Read the model definition and answer for the solid it produces. Units are mm, in the model's axes. A direction names the side the tool comes from. Coordinates: 2 decimals unless noted, no trailing zeros. Write each loop counter-clockwise with the first axis right and the second up, starting at its lowest first coordinate (ties: lowest second). Pieces come first, ordered by that corner, then holes. Notation, with made-up numbers: (-24, -30) -> (23, -30) arc R27 ccw to (23, 2) -> close; hole circle Ø8 at (89.25, 47). An arc over 180 degrees is marked (long way). One line per item, written item: value. Start each with the question number.
from build123d import *

# Parameters (mm, degrees)
RESSALTO_EXTRUS_O1_DEPTH = 5
ESBO_O4_W                = 4.495494134
ESBO_O4_H                = 25
CORTE_EXTRUS_O2_DEPTH    = 5
ESBO_O11_W               = 5
ESBO_O11_H               = 25
CORTE_EXTRUS_O8_DEPTH    = 10
ESBO_O24_W               = 15
ESBO_O24_H               = 60
CORTE_EXTRUS_O14_DEPTH   = 10
ESBO_O27_W               = 15
ESBO_O27_H               = 60
CORTE_EXTRUS_O16_DEPTH   = 25


with BuildPart() as part:
    # Esboço1 → Ressalto-extrusão1 (new body)
    with BuildSketch(Plane.XY):
        with BuildLine():
            Line((-47.810925728, 58.485502959), (65.189074272, 58.485502959))
            ThreePointArc((65.189074272, 58.485502959), (68.724608178, 57.021036865), (70.189074272, 53.485502959))
            Line((70.189074272, 53.485502959), (70.189074272, -59.514497041))
            ThreePointArc((70.189074272, -59.514497041), (68.724608178, -63.050030947), (65.189074272, -64.514497041))
            Line((65.189074272, -64.514497041), (-47.810925728, -64.514497041))
            ThreePointArc((-47.810925728, -64.514497041), (-51.346459634, -63.050030947), (-52.810925728, -59.514497041))
            Line((-52.810925728, -59.514497041), (-52.810925728, 53.485502959))
            ThreePointArc((-52.810925728, 53.485502959), (-51.346459634, 57.021036865), (-47.810925728, 58.485502959))
        make_face()
    extrude(amount=RESSALTO_EXTRUS_O1_DEPTH)

    # Esboço4 → Corte-extrusão2 (cut)
    with BuildSketch(Plane.XY.offset(5)):
        with Locations((-50.563178661, 37.985502959)):
            Rectangle(ESBO_O4_W, ESBO_O4_H)
    extrude(amount=-CORTE_EXTRUS_O2_DEPTH, mode=Mode.SUBTRACT)

    # Esboço11 → Corte-extrusão8 (cut)
    with BuildSketch(Plane.XY.offset(5)):
        with Locations((67.689074272, 37.985502959)):
            Rectangle(ESBO_O11_W, ESBO_O11_H)
    extrude(amount=-CORTE_EXTRUS_O8_DEPTH, mode=Mode.SUBTRACT)

    # Esboço24 → Corte-extrusão14 (cut)
    with BuildSketch(Plane.XY.offset(5)):
        with Locations((-45.310925728, -19.514497041)):
            Rectangle(ESBO_O24_W, ESBO_O24_H)
    extrude(amount=-CORTE_EXTRUS_O14_DEPTH, mode=Mode.SUBTRACT)

    # Esboço27 → Corte-extrusão16 (cut)
    with BuildSketch(Plane.XY.offset(5)):
        with Locations((62.689074272, -19.514497041)):
            Rectangle(ESBO_O27_W, ESBO_O27_H)
    extrude(amount=-CORTE_EXTRUS_O16_DEPTH, mode=Mode.SUBTRACT)


solid = part.part
1. A cutting plane is placed at C-C on y = -26. Give the vertices of the cut face in (x, z), then the cut area to 3 significant figures.
2. For a pull along Z with two mould halves and no side action, classify faces 4 (the face through (10, -2, 0)), 5 (the face through (10, -2, 5)), 6 (the face through (-48.315, 38, 3)) as +Z half, -Z half, draft (parallel to the pull), parting line (faces both ways), or undercut.
3. A cutting plane is placed at B-B on z = 3.4. Give the vertices of the cut face in (x, y).
4. Given pin 1 (1.5 mm diameter, centred on x = 67.5, z = 2, fed in from -Y); pin 2 (4 mm diameter, centred on x = -25, y = 5, fed in from -Z); pin 3 (2.5 mm diameter, centred on y = 38.5, z = 3, fed in from -X); pin 4 (1.3 mm diameter, centred on x = -51.5, z = 3, fed in from -Y), each flat-ended and moving along its own axis, determine where each tip first touches the part or whether it passes through.
5. Find the intervals of material crossed by probe 1 along Y at (x, z) = (-42, 1); probe 2 along X at (y, z) = (-7, 0.4); probe 3 along X at (y, z) = (40.5, 3.4), in increasing order. Write a range as from..to.
6. A tool of negligible diameter and unlimited length cuts with its end or side. For faces 1 (the face through (-45, -49.514, 3)), 2 (the face through (63, -49.514, 3)), 3 (the face through (-51.385, 56.982, 2.465)), from which of +Z, -Z, +X, -X, +Y, -Y can it reach the whole face along a straight path? Write none if from no direction.
7. A cutting plane is placed at A-A on x = 58. Give the vertices of the cut face in (y, z).
Derived:
1. outline: (-37.81, 0) -> (55.19, 0) -> (55.19, 5) -> (-37.81, 5) -> close
1. area: 465 mm2
2. face 4: -Z half
2. face 5: +Z half
2. face 6: draft
3. outline: (-52.81, -59.51) arc R5 ccw to (-47.81, -64.51) -> (65.19, -64.51) arc R5 ccw to (70.19, -59.51) -> (70.19, -49.51) -> (55.19, -49.51) -> (55.19, 10.49) -> (70.19, 10.49) -> (70.19, 25.49) -> (65.19, 25.49) -> (65.19, 50.49) -> (70.19, 50.49) -> (70.19, 53.49) arc R5 ccw to (65.19, 58.49) -> (-47.81, 58.49) arc R5 ccw to (-52.81, 53.49) -> (-52.81, 50.49) -> (-48.32, 50.49) -> (-48.32, 25.49) -> (-52.81, 25.49) -> (-52.81, 10.49) -> (-37.81, 10.49) -> (-37.81, -49.51) -> (-52.81, -49.51) -> close
4. pin 1: stops at y = -64.26
4. pin 2: stops at z = 0
4. pin 3: stops at x = -48.32
4. pin 4: stops at y = -63.48
5. probe 1: y = -64.51..-49.51, 10.49..58.49
5. probe 2: x = -37.81..55.19
5. probe 3: x = -48.32..65.19
6. face 1: +Z, -Z, -X
6. face 2: +Z, -Z, +X
6. face 3: +Z, -Z, -X, +Y
7. outline: (-64.51, 0) -> (-49.51, 0) -> (-49.51, 5) -> (-64.51, 5) -> close; (10.49, 0) -> (58.49, 0) -> (58.49, 5) -> (10.49, 5) -> close
